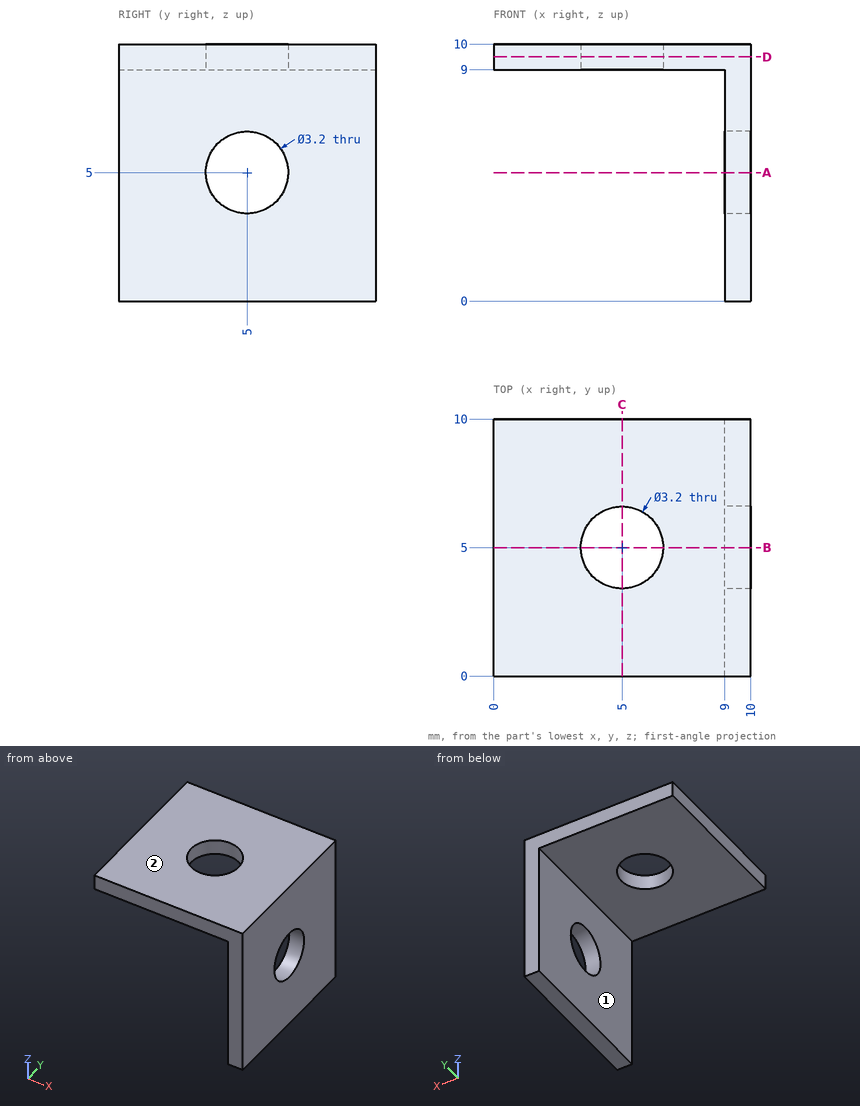
Input: dimensioned drawing with shaded views. Units: mm. Origin: part minimum x, y, z. A direction names the side the tool comes from. Round coordinates to 2 decimals unless told otherwise and drop trailing zeros. Loops run counter-clockwise (first coordinate to the right, second up) from the corner with the lowest first, then second, coordinate; pieces in that order, holes last. Notation, with made-up numbers: M 40.25,81 L 49.25,81 A20 ccw 49.25,106 Z; hole C 0.25,58.25 d6. An arc over 180 degrees is marked long. One line per question, with ' | ' between items.
(1) Cut plane D-D on z = 9.5. Return the cut outline in (x, y), plus the area to 3 significant figures.
Check result:
outline: M 0,0 L 10,0 L 10,10 L 0,10 Z; hole C 5,5 d3.2 | area: 92.0 mm2
(2) Material intervals for line 1 along Z through (x, y) = (9.6, 5); line 2 along X through (y, z) = (7.5, 4), sorted ascending. Write a range as from..to.
Check result:
line 1: z = 0..3.4, 6.6..10 | line 2: x = 9..10
(3) Contact query for flat-ended pins moving along their axis: P1, Ø6, axis at y = 2, z = 8, coming from the -X side; P2, Ø1.5, axis at x = 8, y = 6, coming from the -Z side; P3, Ø3, axis at y = 7.5, z = 3.5, coming from the -X side. Output: stop coordinate, or through.
Check result:
P1: stops at x = 0 | P2: stops at z = 9 | P3: stops at x = 9
(4) Cut plane C-C on x = 5. Return the cut outline in (y, z).
Check result:
outline: M 0,9 L 3.4,9 L 3.4,10 L 0,10 Z; M 6.6,9 L 10,9 L 10,10 L 6.6,10 Z
(5) Access query for the marked faces 1 and 2. Directions: +Z, -Z, +X, -X, +Y, -Y. A direction counts if a zero-diameter tool reaches every point of the face in a straight line with its end or side. Return the directions, or none.
Check result:
face 1: -Z, -X, +Y, -Y | face 2: +Z, +X, -X, +Y, -Y
(6) Cut plane A-A on z = 5. Return the cut outline in (x, y), plus the area to 3 significant figures.
Check result:
outline: M 9,0 L 10,0 L 10,3.4 L 9,3.4 Z; M 9,6.6 L 10,6.6 L 10,10 L 9,10 Z | area: 6.80 mm2
(7) Cut plane B-B on y = 5. Return the cut outline in (x, z), plus the area to 3 significant figures.
Check result:
outline: M 0,9 L 3.4,9 L 3.4,10 L 0,10 Z; M 6.6,9 L 9,9 L 9,6.6 L 10,6.6 L 10,10 L 6.6,10 Z; M 9,0 L 10,0 L 10,3.4 L 9,3.4 Z | area: 12.6 mm2
